from build123d import *

# Parameters (mm, degrees)
BOSS_EXTRUDE1_DEPTH    = 1.5875
F_10_CLEARANCE_HOLE1_D = 5.6134
SKETCH5_R              = 14.2875
CUT_EXTRUDE1_DEPTH     = 448.730108977


with BuildPart() as part:
    # Sketch1 → Boss-Extrude1 (new body)
    with BuildSketch(Plane.XY):
        Polygon((0, 0), (0, 203.2), (398.960512242, 68.760512242), (398.960512242, 17.960512242), (68.760512242, 17.960512242), (50.8, 0), align=None)
    extrude(amount=BOSS_EXTRUDE1_DEPTH)

    # #10 Clearance Hole1 (through all)
    with Locations(Plane(origin=(0, 0, 0), x_dir=(-1, 0, 0), z_dir=(0, 0, -1))):
        with Locations((-12.7, 102.542512242), (-22.225, 76.573552108), (-22.225, 10.147472376)):
            Hole(F_10_CLEARANCE_HOLE1_D / 2)

    # Sketch5 → Cut-Extrude1 (cut, through all)
    with BuildSketch(Plane.XY.offset(1.5875)):
        with Locations((63.5, 106.860512242)):
            Circle(SKETCH5_R)
    extrude(amount=-CUT_EXTRUDE1_DEPTH, mode=Mode.SUBTRACT)


solid = part.part
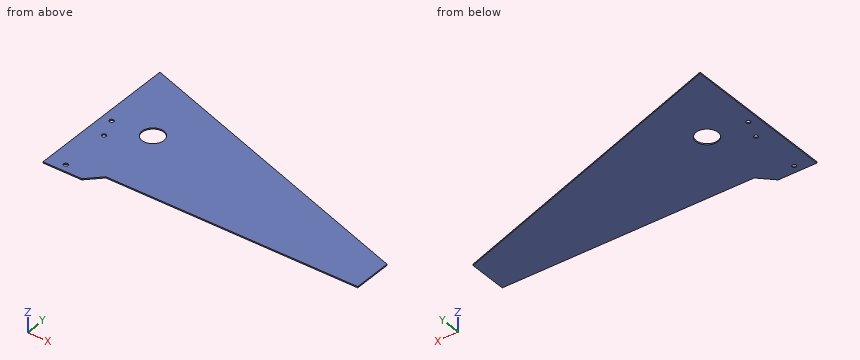
Verification items for the finished model (mm, model axes). Coordinates: 2 decimals unless noted, no trailing zeros. Write each loop counter-clockwise with the first axis right and the second up, starting at its lowest first coordinate (ties: lowest second). Pieces come first, ordered by that corner, then holes. Notation, with made-up numbers: M 81,-6.75 L 139,-6.75 A24 cw 139,17.25 Z; hole C 19.5,25.25 d3. An arc over 180 degrees is marked long. Use a Markdown table: item, result.
Q1. Sectioned sample at A-A, the plane y = 117. Record the boundary of the cut face in (x, z), plus the area to 3 significant figures.
Reply:
| item | result |
|---|---|
| outline | M 0,0 L 53.43,0 L 53.43,1.59 L 0,1.59 Z; M 73.57,0 L 255.81,0 L 255.81,1.59 L 73.57,1.59 Z |
| area | 374 mm² |
Q2. Go/stop test with flat-tipped pins: P1, Ø5, axis at x = 22.22, y = 10.15, coming from the -Z side; P2, Ø0.8, axis at x = 244.5, z = 0.5, coming from the -Y side. Record where each tip stops, or that it passes through.
Reply:
| item | result |
|---|---|
| P1 | passes through |
| P2 | stops at y = 17.96 |
Q3. Sectioned sample at B-B, the plane z = 0.9. Record the boundary of the cut face in (x, y) (1 decimal).
Reply:
| item | result |
|---|---|
| outline | M 0,0 L 50.8,0 L 68.8,18 L 399,18 L 399,68.8 L 0,203.2 Z; hole C 12.7,102.5 d5.6; hole C 22.2,10.1 d5.6; hole C 22.2,76.6 d5.6; hole C 63.5,106.9 d28.6 |
Q4. Sectioned sample at C-C, the plane x = 63.5. Record the boundary of the cut face in (y, z), plus the area to 3 significant figures.
Reply:
| item | result |
|---|---|
| outline | M 12.7,0 L 92.57,0 L 92.57,1.59 L 12.7,1.59 Z; M 121.15,0 L 181.8,0 L 181.8,1.59 L 121.15,1.59 Z |
| area | 223 mm² |
Q5. Sectioned sample at D-D, the plane y = 165. Record the boundary of the cut face in (x, z), plus the area to 3 significant figures.
Reply:
| item | result |
|---|---|
| outline | M 0,0 L 113.36,0 L 113.36,1.59 L 0,1.59 Z |
| area | 180 mm² |
Q6. Thickness scan on line 1 (Y direction, x = 21.5, z = 0.75) (3 decimals); line 2 (Y direction, x = 12.7, z = 1.1); line 3 (Y direction, x = 63.5, z = 0.85). Record the ranges inside material, lowest first.
Reply:
| item | result |
|---|---|
| line 1 | y = 0 to 7.436, 12.859 to 73.862, 79.285 to 195.955 |
| line 2 | y = 0 to 99.74, 105.35 to 198.92 |
| line 3 | y = 12.7 to 92.57, 121.15 to 181.8 |
